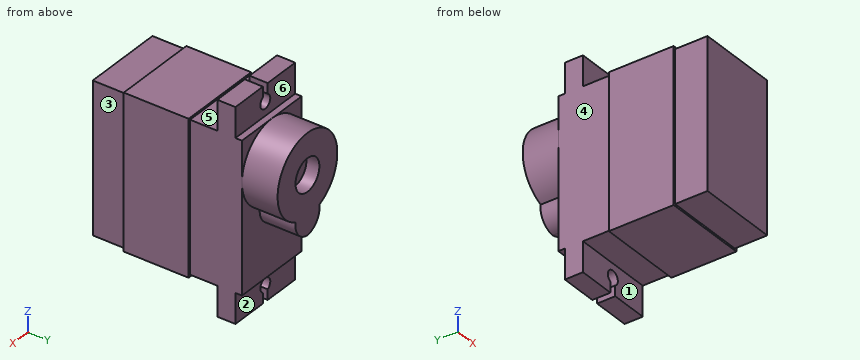
Autodesk Inventor part; units mm, degrees
ref_plane "YZ Plane" through (0, 0, 0) normal (1, 0, 0) x (0, 1, 0)
ref_plane "XZ Plane" through (0, 0, 0) normal (0, 1, 0) x (-1, 0, 0)
ref_plane "XY Plane" through (0, 0, 0) normal (0, 0, 1) x (1, 0, 0)
sketch "Sketch1" plane through (0, 0, 0) normal (0, 1, 0) x (-1, 0, 0)
  line L0 (0, 0) -> (12.5, 0)
  line L1 (12.5, 0) -> (12.5, 23)
  line L2 (12.5, 23) -> (0, 23)
  line L3 (0, 23) -> (0, 0)
  dimension "d0" = 12.5
  dimension "d1" = 23
extrude "Extrusion1" add sketch "Sketch1" along normal blind 23
sketch "Sketch2" plane through (0, 23, 0) normal (0, 1, 0) x (1, 0, 0)
  line L0 (0, 0) -> (-12.5, 0)
  line L1 (-12.5, 0) -> (-12.5, -23)
  line L2 (-12.5, -23) -> (0, -23)
  line L3 (0, -23) -> (0, 0)
  line L4 (0, 4.6) -> (-12.5, 4.6)
  line L5 (-12.5, 4.6) -> (-12.5, -27.6)
  line L6 (-12.5, -27.6) -> (0, -27.6)
  line L7 (0, -27.6) -> (0, 4.6)
  line L8 (0, 4.6) -> (-12.5, -27.6) construction
  line L9 (-12.5, 4.6) -> (0, -27.6) construction
  point P0 (-6.25, -11.5)
  dimension "d4" = 32.2
extrude "Extrusion2" add sketch "Sketch2" against normal blind 3.8 contours L0 L5 L4 L7 | L7 L6 L5 L2
sketch "Sketch3" plane through (0, 23, 0) normal (0, 1, 0) x (1, 0, 0)
  line L0 (-12.5, 4.6) -> (-12.5, -27.6)
  line L1 (-12.5, -27.6) -> (0, -27.6)
  line L2 (0, -27.6) -> (0, 4.6)
  line L3 (0, 4.6) -> (-12.5, 4.6)
  line L4 (0, -23) -> (-12.5, -23)
  line L5 (-12.5, 0) -> (0, 0)
extrude "Extrusion3" cut sketch "Sketch3" against normal blind 1 contours L3 L2 L5 L0 | L4 L2 L1 L0
sketch "Sketch4" plane through (0, 23, 0) normal (0, 1, 0) x (1, 0, 0)
  line L0 (-12.5, -23) -> (0, -23)
  line L1 (-6.25, -23) -> (-6.25, -16.75)
  circle A0 centre (-6.25, -16.75) radius 6.25
  dimension "d9" = 6.25
extrude "Extrusion4" add sketch "Sketch4" along normal blind 5.5
sketch "Sketch5" plane through (-6.25, 28.5, 16.75) normal (0, 1, 0) x (1, 0, 0)
  circle A0 centre (0, 0) radius 6.25
  arc A1 (0, -8.95) -> (2.5, -5.72822) centre (-0.266089, -6.162672) ccw
  arc A2 (-2.5, -5.72822) -> (0, -8.95) centre (0.266089, -6.162672) ccw
  arc A3 (0, -8.95) -> (2.5, -5.72822) centre (-0.266089, -6.162672) ccw
  arc A4 (-2.5, -5.72822) -> (0, -8.95) centre (0.266089, -6.162672) ccw
  arc A5 (-2.5, -5.72822) -> (2.5, -5.72822) centre (0, 0) ccw
  line L0 (0, 0) -> (-2.287713, 0)
  arc A6 (2.5, 5.72822) -> (0, 8.95) centre (-0.266089, 6.162672) ccw
  arc A7 (0, 8.95) -> (-2.5, 5.72822) centre (0.266089, 6.162672) ccw
  arc A8 (2.5, 5.72822) -> (0, 8.95) centre (-0.266089, 6.162672) ccw
  arc A9 (0, 8.95) -> (-2.5, 5.72822) centre (0.266089, 6.162672) ccw
  arc A10 (2.5, 5.72822) -> (-2.5, 5.72822) centre (0, 0) ccw
  point P0 (6.25, 16.75)
  dimension "d14" = 2.8
extrude "Extrusion5" add sketch "Sketch5" against normal blind 7.5 contours A0 A7 A6
sketch "Sketch6" plane through (0, 28.5, 0) normal (0, 1, 0) x (1, 0, 0)
  arc A0 (-8.75, -11.02178) -> (-3.75, -11.02178) centre (-6.25, -16.75) ccw
  circle A1 centre (-6.25, -16.75) radius 3.475
  point P0 (0, 0)
  dimension "d17" = 6.95
extrude "Extrusion6" cut sketch "Sketch6" against normal blind 2
sketch "Sketch7" plane through (0, 28.5, 0) normal (0, 1, 0) x (1, 0, 0)
  circle A0 centre (-6.25, -16.75) radius 3.475
  arc A1 (-8.75, -11.02178) -> (-3.75, -11.02178) centre (-6.25, -16.75) ccw
  circle A2 centre (-6.25, -16.75) radius 3.5
  point P0 (0, 0)
  dimension "d20" = 7
sketch "Sketch7 outline for Extrusion7" plane through (0, 28.5, 0) normal (0, 1, 0) x (1, 0, 0)
  circle A0 centre (-6.25, -16.75) radius 3.475
extrude "Extrusion7" cut sketch "Sketch7 outline for Extrusion7" against normal blind 2
sketch "Sketch8" plane through (0, 22, 0) normal (0, 1, 0) x (1, 0, 0)
  line L0 (0, -27.6) -> (-12.5, -27.6)
  line L1 (0, -23) -> (0, -27.6)
  line L2 (-12.5, -23) -> (0, -23)
  line L3 (-12.5, -27.6) -> (-12.5, -23)
  line L4 (-12.5, 0) -> (-12.5, 4.6)
  line L5 (0, 0) -> (-12.5, 0)
  line L6 (0, 4.6) -> (0, 0)
  line L7 (-12.5, 4.6) -> (0, 4.6)
  arc A0 (-5.75, -26.013179) -> (-6.75, -26.013179) centre (-6.25, -25.1) ccw
  arc A1 (-6.75, -27.6) -> (-5.75, -27.6) centre (-6.25, -27.6) ccw
  line L8 (0, -27.6) -> (-12.5, -27.6)
  line L9 (-5.75, -27.6) -> (-5.75, -26.013179)
  line L10 (-6.75, -27.6) -> (-6.75, -26.013179)
  line L11 (0, -23) -> (0, 0)
  line L12 (0, -11.5) -> (-20.862921, -11.5)
  arc A2 (-6.75, 3.013179) -> (-5.75, 3.013179) centre (-6.25, 2.1) ccw
  arc A3 (-5.75, 4.6) -> (-6.75, 4.6) centre (-6.25, 4.6) ccw
  line L13 (-5.75, 4.6) -> (-5.75, 3.013179)
  line L14 (-6.75, 4.6) -> (-6.75, 3.013179)
extrude "Extrusion8" cut sketch "Sketch8" against normal blind 10 contours L0 L10 A0 L9 | A3 L7 | L7 L13 A2 L14
sketch "Sketch9" plane through (0, 28.5, 0) normal (0, 1, 0) x (1, 0, 0)
  circle A0 centre (-6.25, -16.75) radius 3.475
  arc A1 (-8.75, -11.02178) -> (-3.75, -11.02178) centre (-6.25, -16.75) ccw
  arc A2 (-3.75, -11.02178) -> (-6.25, -7.8) centre (-6.516089, -10.587328) ccw
  arc A3 (-6.25, -7.8) -> (-8.75, -11.02178) centre (-5.983911, -10.587328) ccw
  circle A4 centre (-6.25, -16.75) radius 2.5
  point P0 (0, 0)
  dimension "d29" = 5
extrude "Extrusion9" add sketch "Sketch9" against normal blind 10 contours A0
sketch "Sketch10" plane through (-12.5, 0, 0) normal (-1, 0, 0) x (0, 0, 1)
  line L0 (0, 23) -> (0, 22)
  line L1 (0, 22) -> (-4.6, 22)
  line L2 (-4.6, 22) -> (-4.6, 19.2)
  line L3 (0, 19.2) -> (-4.6, 19.2)
  line L4 (0, 0) -> (0, 19.2)
  line L5 (0, 0) -> (23, 0)
  line L6 (23, 0) -> (23, 19.2)
  line L7 (27.6, 19.2) -> (23, 19.2)
  line L8 (27.6, 22) -> (27.6, 19.2)
  line L9 (27.6, 22) -> (23, 22)
  line L10 (23, 22) -> (23, 23)
  line L11 (16.75, 23) -> (23, 23)
  line L12 (0, 23) -> (16.75, 23)
  line L13 (0, 0) -> (0, 5)
  line L14 (0, 0) -> (0, 19.2)
  line L15 (0, 5) -> (23, 5)
  line L16 (23, 0) -> (23, 19.2)
  line L17 (0, 5) -> (0, 15)
  line L18 (0, 15) -> (23, 15)
  dimension "d32" = 5
  dimension "d33" = 10
extrude "Extrusion11" add sketch "Sketch10" along normal blind 0.3 contours L18 L6 L15 L4
sketch "Sketch11" plane through (-12.5, 0, 23) normal (0, 0, 1) x (1, 0, 0)
  line L0 (12.5, 0) -> (12.5, 19.2)
  line L1 (-0.3, 5) -> (-0.3, 15)
  line L2 (-0.3, 15) -> (12.5, 15)
  line L3 (12.5, 15) -> (12.8, 15)
  line L4 (12.8, 15) -> (-0.3, 15)
  line L5 (-0.3, 15) -> (-0.3, 5)
  line L6 (-0.3, 5) -> (12.8, 5)
  line L7 (12.8, 5) -> (12.8, 15)
  point P0 (0, 15)
  dimension "d38" = 0.3
extrude "Extrusion12" add sketch "Sketch11" along normal blind 0.3
sketch "Sketch12" plane through (0, 0, 23) normal (1, 0, 0) x (0, 0, -1)
  line L0 (23, 22) -> (23, 23)
  line L1 (6.25, 23) -> (23, 23)
  line L2 (0, 23) -> (6.25, 23)
  line L3 (0, 23) -> (0, 22)
  line L4 (0, 22) -> (-4.6, 22)
  line L5 (-4.6, 22) -> (-4.6, 19.2)
  line L6 (0, 19.2) -> (-4.6, 19.2)
  line L7 (0, 15) -> (0, 19.2)
  line L8 (0, 5) -> (0, 15)
  line L9 (0, 0) -> (0, 5)
  line L10 (0, 0) -> (23, 0)
  line L11 (23, 0) -> (23, 19.2)
  line L12 (27.6, 19.2) -> (23, 19.2)
  line L13 (27.6, 22) -> (27.6, 19.2)
  line L14 (27.6, 22) -> (23, 22)
  line L15 (23, 0) -> (23, 19.2)
  line L16 (-0.411339, 5) -> (23, 5)
  line L17 (23, 5) -> (23.3, 5)
  line L18 (-0.3, 15) -> (23.3, 15)
  line L19 (23.3, 15) -> (23.3, 5)
  line L20 (23.3, 5) -> (-0.3, 5)
  line L21 (-0.3, 5) -> (-0.3, 15)
  dimension "d41" = 0.3
extrude "Extrusion13" add sketch "Sketch12" along normal blind 0.3 contours L18 L19 L17 L11 | L11 L16 L8 L18 | L8 L16 L21 L18
sketch "Sketch13" plane through (0, 0, 0) normal (0, 0, -1) x (-1, 0, 0)
  line L0 (-0.3, 5) -> (12.8, 5)
  line L1 (12.8, 5) -> (12.8, 15)
  line L2 (12.8, 15) -> (-0.3, 15)
  line L3 (-0.3, 15) -> (-0.3, 5)
  point P0 (0, 0)
extrude "Extrusion14" add sketch "Sketch13" along normal blind 0.3
properties part number "servo" material "LCP Plastic"
Model file for the job. Use its own axes, mm. Face numbers are marked on the shaded views. A direction names the side the tool comes from. Give positions to 0.01 mm unless a question says otherwise; leave off trailing zeros. Loops run counter-clockwise (first coordinate to the right, second up) from the corner with the lowest first, then second, coordinate; pieces in that order, holes last. Notation, with made-up numbers: (-38.75, 45.5) -> (-25.75, 45.5) arc R19 ccw to (-25.75, 64.5) -> close; hole circle Ø10 at (72, 45). An arc over 180 degrees is marked (long way). Use a Markdown table: item, result. Add a question column.
(1) Mould opens along Y. For the marked faces 4, 5 and 6 say: +Y half, -Y half, draft (parallel to the pull), parting line (faces both ways), or undercut.
(2) Tool access for the marked faces 1, 2 and 3: list every direction of +Z, -Z, +X, -X, +Y, -Y with a clear straight run to the whole face (end or side of a thin tool).
(3) Wall check: line 1 along Z through (x, y) = (-6.25, 27.7); line 2 along X through (y, z) = (20.7, 25.1); line 3 along Z through (x, y) = (-8.25, 7.75). Give the ranges that are in metal, low to high.
(4) Drop flat-ended pins along their axis: pin 1 Ø3.5 at (x, z) = (-3.5, 25.5) entering from +Y; pin 2 Ø4 at (y, z) = (17.5, 10) entering from -X; pin 3 Ø1 at (x, y) = (-4.5, 17.5) entering from +Z. Give the stop position or say it passes through.
(5) Slice it at C-C on x = -12. List the corners of the cut face in (y, z), and give its area (3 significant figures).
(6) Slice it at A-A on z = 25.1. List the corners of the cut face in (x, y), and give its area (3 significant figures).
(7) Slice it at D-D on y = 13. List the corners of the cut face in (x, z), and give its area (3 significant figures).
(8) Slice it at B-B on z = 1.5. List the corners of the cut face in (x, y), and give its area (4 significant figures).
Filled sheet:
| question | item | result |
|---|---|---|
| 1 | face 4 | draft |
| 1 | face 5 | undercut |
| 1 | face 6 | +Y half |
| 2 | face 1 | -Z, +X, -X |
| 2 | face 2 | -Z, +X, -X, +Y |
| 2 | face 3 | +Z, -Z, +X, -Y |
| 3 | line 1 | 7.8 to 14.25, 19.25 to 23 |
| 3 | line 2 | -12.5 to -7.29, -5.21 to 0 |
| 3 | line 3 | -0.3 to 23.3 |
| 4 | pin 1 | y = 22 |
| 4 | pin 2 | x = -12.5 |
| 4 | pin 3 | z = 23 |
| 5 | outline | (0, 0) -> (5, 0) -> (5, -0.3) -> (15, -0.3) -> (15, 0) -> (19.2, 0) -> (19.2, -4.6) -> (22, -4.6) -> (22, 0) -> (23, 0) -> (23, 14.3) -> (28.5, 14.3) -> (28.5, 19.2) -> (23, 19.2) -> (23, 23) -> (22, 23) -> (22, 27.6) -> (19.2, 27.6) -> (19.2, 23) -> (15, 23) -> (15, 23.3) -> (5, 23.3) -> (5, 23) -> (0, 23) -> close |
| 5 | area | 588 mm2 |
| 6 | outline | (-12.5, 19.2) -> (-7.29, 19.2) -> (-7.29, 22) -> (-12.5, 22) -> close; (-5.21, 19.2) -> (0, 19.2) -> (0, 22) -> (-5.21, 22) -> close |
| 6 | area | 29.2 mm2 |
| 7 | outline | (-12.8, -0.3) -> (0.3, -0.3) -> (0.3, 23.3) -> (-12.8, 23.3) -> close |
| 7 | area | 309 mm2 |
| 8 | outline | (-12.8, 5) -> (-12.5, 5) -> (-12.5, 0) -> (0, 0) -> (0, 5) -> (0.3, 5) -> (0.3, 15) -> (0, 15) -> (0, 23) -> (-12.5, 23) -> (-12.5, 15) -> (-12.8, 15) -> close |
| 8 | area | 293.5 mm2 |
